from build123d import *

# Parameters (mm, degrees)
Y_KSEKLIK_EKSTR_ZYON3_DEPTH = 3
KES_EKSTR_ZYON10_DEPTH      = 3
KES_EKSTR_ZYON11_DEPTH      = 3
KES_EKSTR_ZYON14_DEPTH      = 3
KES_EKSTR_ZYON15_DEPTH      = 3
IZIM25_R                    = 1.6
KES_EKSTR_ZYON16_DEPTH      = 10
IZIM33_R                    = 2.1
IZIM33_R_2                  = 1.6
KES_EKSTR_ZYON18_DEPTH      = 3
IZIM34_R                    = 1.6
KES_EKSTR_ZYON19_DEPTH      = 10
KES_EKSTR_ZYON21_DEPTH      = 10
IZIM38_R                    = 1.5
KES_EKSTR_ZYON22_DEPTH      = 10
IZIM39_W                    = 25
IZIM39_H                    = 9
KES_EKSTR_ZYON23_DEPTH      = 10
IZIM40_R                    = 1.6
KES_EKSTR_ZYON24_DEPTH      = 100


with BuildPart() as part:
    # Çizim16 → Yükseklik-Ekstrüzyon3 (new body)
    with BuildSketch(Plane(origin=(0, 0, 0), x_dir=(1, 0, 0), z_dir=(0, 1, 0))):
        with BuildLine():
            Line((-110, -70), (100, -70))
            ThreePointArc((100, -70), (107.071067812, -67.071067812), (110, -60))
            Line((110, -60), (110, 60))
            ThreePointArc((110, 60), (107.071067812, 67.071067812), (100, 70))
            Line((100, 70), (-110, 70))
            Line((-110, 70), (-110, -70))
        make_face()
    extrude(amount=Y_KSEKLIK_EKSTR_ZYON3_DEPTH)

    # Çizim18 → Kes-Ekstrüzyon10 (cut)
    with BuildSketch(Plane(origin=(0, 3, 0), x_dir=(1, 0, 0), z_dir=(0, 1, 0))):
        with BuildLine():
            Line((-19, 70), (-25.463821511, 59.889658192))
            ThreePointArc((-25.463821511, 59.889658192), (-43.144058736, 50.67991016), (-60, 61.323569832))
            ThreePointArc((-60, 61.323569832), (-63.804672609, 66.383043129), (-69, 70))
            Line((-69, 70), (-19, 70))
        make_face()
    extrude(amount=-KES_EKSTR_ZYON10_DEPTH, mode=Mode.SUBTRACT)

    # Çizim19 → Kes-Ekstrüzyon11 (cut)
    with BuildSketch(Plane(origin=(0, 3, 0), x_dir=(1, 0, 0), z_dir=(0, 1, 0))):
        with BuildLine():
            Line((-19, -70), (-25.463821511, -59.889658192))
            ThreePointArc((-25.463821511, -59.889658192), (-43.144058736, -50.67991016), (-60, -61.323569832))
            ThreePointArc((-60, -61.323569832), (-63.804672609, -66.383043129), (-69, -70))
            Line((-69, -70), (-19, -70))
        make_face()
    extrude(amount=-KES_EKSTR_ZYON11_DEPTH, mode=Mode.SUBTRACT)

    # Çizim23 → Kes-Ekstrüzyon14 (cut)
    with BuildSketch(Plane(origin=(0, 3, 0), x_dir=(1, 0, 0), z_dir=(0, 1, 0))):
        with BuildLine():
            Line((-84, -70), (-90.329717397, -53.149638649))
            ThreePointArc((-90.329717397, -53.149638649), (-98.077113424, -40.633105793), (-110, -32))
            Line((-110, -32), (-110, -70))
            Line((-110, -70), (-84, -70))
        make_face()
    extrude(amount=-KES_EKSTR_ZYON14_DEPTH, mode=Mode.SUBTRACT)

    # Çizim24 → Kes-Ekstrüzyon15 (cut)
    with BuildSketch(Plane(origin=(0, 3, 0), x_dir=(1, 0, 0), z_dir=(0, 1, 0))):
        with BuildLine():
            Line((-84, 70), (-90.329717397, 53.149638649))
            ThreePointArc((-90.329717397, 53.149638649), (-98.077113424, 40.633105793), (-110, 32))
            Line((-110, 32), (-110, 70))
            Line((-110, 70), (-84, 70))
        make_face()
    extrude(amount=-KES_EKSTR_ZYON15_DEPTH, mode=Mode.SUBTRACT)

    # Çizim25 → Kes-Ekstrüzyon16 (cut)
    with BuildSketch(Plane(origin=(0, 3, 0), x_dir=(1, 0, 0), z_dir=(0, 1, 0))):
        with Locations(Location((-95, 28, 0), (0, 0, 270))):
            Circle(IZIM25_R)
        with Locations(Location((-95, -28, 0), (0, 0, 270))):
            Circle(IZIM25_R)
    extrude(amount=-KES_EKSTR_ZYON16_DEPTH, mode=Mode.SUBTRACT)

    # Çizim33 → Kes-Ekstrüzyon18 (cut)
    with BuildSketch(Plane(origin=(0, 3, 0), x_dir=(1, 0, 0), z_dir=(0, 1, 0))):
        with Locations(Location((-75, -60, 0), (0, 0, 270))):
            Circle(IZIM33_R)
        with Locations(Location((-75, 60, 0), (0, 0, 270))):
            Circle(IZIM33_R)
        with Locations(Location((-75, 45, 0), (0, 0, 270))):
            Circle(IZIM33_R_2)
        with Locations(Location((-75, -45, 0), (0, 0, 270))):
            Circle(IZIM33_R_2)
    extrude(amount=-KES_EKSTR_ZYON18_DEPTH, mode=Mode.SUBTRACT)

    # Çizim34 → Kes-Ekstrüzyon19 (cut)
    with BuildSketch(Plane(origin=(0, 3, 0), x_dir=(1, 0, 0), z_dir=(0, 1, 0))):
        with Locations(Location((95, -65, 0), (0, 0, 270))):
            Circle(IZIM34_R)
        with Locations(Location((95, 65, 0), (0, 0, 270))):
            Circle(IZIM34_R)
    extrude(amount=-KES_EKSTR_ZYON19_DEPTH, mode=Mode.SUBTRACT)

    # Çizim37 → Kes-Ekstrüzyon21 (cut)
    with BuildSketch(Plane(origin=(0, 3, 0), x_dir=(1, 0, 0), z_dir=(0, 1, 0))):
        with BuildLine():
            Line((-73.628967409, -20.666004446), (-37.018589471, -20.666004446))
            ThreePointArc((-37.018589471, -20.666004446), (-29.947521659, -17.737072258), (-27.018589471, -10.666004446))
            Line((-27.018589471, -10.666004446), (-27.018589471, 16.938177002))
            ThreePointArc((-27.018589471, 16.938177002), (-29.947521659, 24.009244814), (-37.018589471, 26.938177002))
            Line((-37.018589471, 26.938177002), (-73.628967409, 26.938177002))
            ThreePointArc((-73.628967409, 26.938177002), (-80.700035221, 24.009244814), (-83.628967409, 16.938177002))
            Line((-83.628967409, 16.938177002), (-83.628967409, -10.666004446))
            ThreePointArc((-83.628967409, -10.666004446), (-80.700035221, -17.737072258), (-73.628967409, -20.666004446))
        make_face()
    extrude(amount=-KES_EKSTR_ZYON21_DEPTH, mode=Mode.SUBTRACT)

    # Çizim38 → Kes-Ekstrüzyon22 (cut)
    with BuildSketch(Plane(origin=(0, 3, 0), x_dir=(1, 0, 0), z_dir=(0, 1, 0))):
        with Locations(Location((57, -58, 0), (0, 0, 270))):
            Circle(IZIM38_R)
        with Locations(Location((82, -58, 0), (0, 0, 270))):
            Circle(IZIM38_R)
        with Locations(Location((57, 58, 0), (0, 0, 270))):
            Circle(IZIM38_R)
        with Locations(Location((82, 58, 0), (0, 0, 270))):
            Circle(IZIM38_R)
    extrude(amount=-KES_EKSTR_ZYON22_DEPTH, mode=Mode.SUBTRACT)

    # Çizim39 → Kes-Ekstrüzyon23 (cut)
    with BuildSketch(Plane(origin=(0, 3, 0), x_dir=(1, 0, 0), z_dir=(0, 1, 0))):
        with Locations((69.5, -65.5)):
            Rectangle(IZIM39_W, IZIM39_H)
        Polygon((57, -70), (57, -61), (39.139428901, -70), align=None)
        Polygon((99.860571099, -70), (82, -61), (82, -70), align=None)
        Polygon((57, 61), (57, 70), (39.139428901, 70), align=None)
        with Locations((69.5, 65.5)):
            Rectangle(IZIM39_W, IZIM39_H)
        Polygon((99.860571099, 70), (82, 70), (82, 61), align=None)
    extrude(amount=-KES_EKSTR_ZYON23_DEPTH, mode=Mode.SUBTRACT)

    # Çizim40 → Kes-Ekstrüzyon24 (cut)
    with BuildSketch(Plane(origin=(0, 3, 0), x_dir=(-1, 0, 0), z_dir=(0, 1, 0))):
        with Locations(Location((-6, -44.857008165, 0), (0, 0, 90))):
            Circle(IZIM40_R)
        with Locations(Location((-50, -46.144414684, 0), (0, 0, 90))):
            Circle(IZIM40_R)
        with Locations(Location((-50, -33.144414684, 0), (0, 0, 90))):
            Circle(IZIM40_R)
        with Locations(Location((-6, -31.857008165, 0), (0, 0, 90))):
            Circle(IZIM40_R)
        with Locations(Location((-50, -20.144414684, 0), (0, 0, 90))):
            Circle(IZIM40_R)
        with Locations(Location((-6, -18.857008165, 0), (0, 0, 90))):
            Circle(IZIM40_R)
    extrude(amount=-KES_EKSTR_ZYON24_DEPTH, mode=Mode.SUBTRACT)


solid = part.part
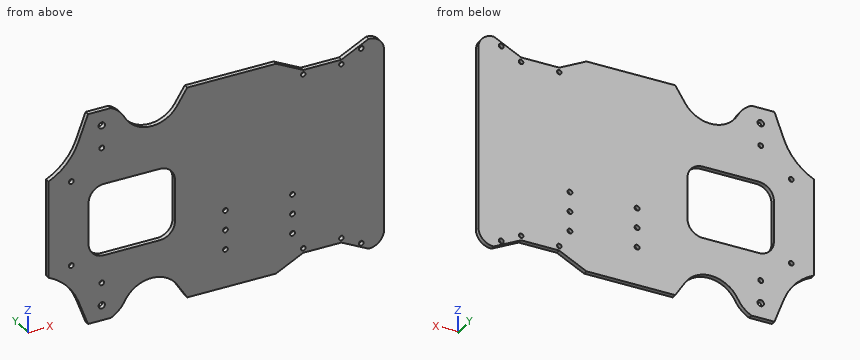
Check sheet for the modelled part. Datum: model origin and axes. Units: mm. Coordinates: 2 decimals unless noted, no trailing zeros. Write each loop counter-clockwise with the first axis right and the second up, starting at its lowest first coordinate (ties: lowest second). Pieces come first, ordered by that corner, then holes. Notation, with made-up numbers: M 35,-6 L 61,-6 A11 ccw 61,13 Z; hole C 15.25,-24 d11. An arc over 180 degrees is marked long. Answer as CSV lines item,"result".
Q1. Go/stop test with flat-tipped pins: pin 1 (3 mm diameter, centred on x = 6, z = -31.86, fed in from +Y); pin 2 (1.5 mm diameter, centred on x = 73, y = 2, fed in from -Z). Record where each tip stops, or that it passes through.
Check result:
pin 1,"through"
pin 2,"z = -61"
Q2. Cross-section at C-C (x = 70). Record the boundary of the cut face in (y, z).
Check result:
outline,"M 0,-61 L 3,-61 L 3,61 L 0,61 Z"
Q3. Cross-section at B-B (y = 2.05). Count the separate pieces of the cut face and the enclosed holes in it, then the cut area to 3 significant figures.
Check result:
separate pieces,"1"
enclosed holes,"19"
area,"24,700 mm^2"
Q4. Cross-section at D-D (x = 46). Record the boundary of the cut face in (y, z).
Check result:
outline,"M 0,-66.54 L 3,-66.54 L 3,66.54 L 0,66.54 Z"
Q5. Cross-section at A-A (z = -8). Record the boundary of the cut face in (x, y).
Check result:
outline,"M -110,0 L -83.63,0 L -83.63,3 L -110,3 Z; M -27.02,0 L 110,0 L 110,3 L -27.02,3 Z"
Q6. Material ranges on probe 1 along Z at (x, y) = (82, 0.9); probe 2 along X at (y, z) = (0.25, -12); probe 3 along Z at (x, y) = (94.5, 2.2), recorded low to high. Write a range as from..to.
Check result:
probe 1,"-61..-59.5, -56.5..56.5, 59.5..61"
probe 2,"-110..-83.63, -27.02..110"
probe 3,"-67.3..-66.52, -63.48..63.48, 66.52..67.3"
